Design review of the part built by this model. Coordinates are the model's own, in mm. Face numbers are marked on the shaded views. Coordinates: 2 decimals unless noted, no trailing zeros. Write each loop counter-clockwise with the first axis right and the second up, starting at its lowest first coordinate (ties: lowest second). Pieces come first, ordered by that corner, then holes.
Q1. Take a section at C-C (x = 0). Give the boundary of the cut face in (y, z) (3 decimals), and give its area (3 significant figures).
Q2. Insertion check: pin 1 (3 mm diameter, centred on x = 23.81, y = 0, fed in from +Z). The pin has a flat end and moves straight along its axis. Give the tip position at first contact, or say it passes through.
Q3. Mouldability with a two-part tool opening along X and no side actions: class the marked faces 1, 2, 3 and 4 as pulls with the +X half, pulls with the -X half, needs draft (parallel to the pull), parting line crosses it, or undercut.
Q4. Take a section at B-B (y = 0). Give the boundary of the cut face in (x, z) (3 decimals).
Q5. Take a section at A-A (z = 1.6). Give the boundary of the cut face in (x, y), and give its area (3 significant figures).
Q6. Take a section at D-D (x = 24). Give the boundary of the cut face in (y, z) (3 decimals), and give its area (3 significant figures).
Q7. For probe 1 along Y at (x, z) = (-22, 0.55); probe 2 along X at (y, z) = (-1.5, 0.85); probe 3 along X at (y, z) = (1.75, 1.5), list the stretches that pass through material, from the lowest coordinate up.
Autodesk Inventor part; units mm, degrees
ref_plane "YZ Plane" through (0, 0, 0) normal (1, 0, 0) x (0, 1, 0)
ref_plane "XZ Plane" through (0, 0, 0) normal (0, 1, 0) x (-1, 0, 0)
ref_plane "XY Plane" through (0, 0, 0) normal (0, 0, 1) x (1, 0, 0)
sketch "Sketch1" plane through (0, 0, 0) normal (0, 0, 1) x (1, 0, 0)
  circle A0 centre (0, 0) radius 23.8125 construction
  circle A1 centre (-23.8125, 0) radius 2.4892
  circle A2 centre (23.8125, 0) radius 2.4892
  line L0 (-23.8125, 0) -> (23.8125, 0) construction
  circle A3 centre (0, 0) radius 2.4892
  arc A4 (-25.4861, 5.4113) -> (-25.4861, -5.4113) centre (-23.8125, 0) ccw
  arc A5 (25.4861, -5.4113) -> (25.4861, 5.4113) centre (23.8125, 0) ccw
  line L1 (-25.4861, 5.4113) -> (-3.7524, 12.133)
  line L2 (3.7524, 12.133) -> (25.4861, 5.4113)
  line L3 (25.4861, -5.4113) -> (3.7524, -12.133)
  line L4 (-3.7524, -12.133) -> (-25.4861, -5.4113)
  arc A6 (-3.7524, -12.133) -> (3.7524, -12.133) centre (0, 0) ccw
  arc A7 (3.7524, 12.133) -> (-3.7524, 12.133) centre (0, 0) ccw
  dimension "d0" = 47.625
  dimension "d1" = 4.9784
  dimension "d2" = 3.175
  dimension "d4" = 12.7
  dimension "d5" = 12.7
extrude "Extrusion1" add sketch "Sketch1" along normal blind 3.175
properties part number "Pison Shaft Replacement Screw Plate" material "Thermoplastic Resin"
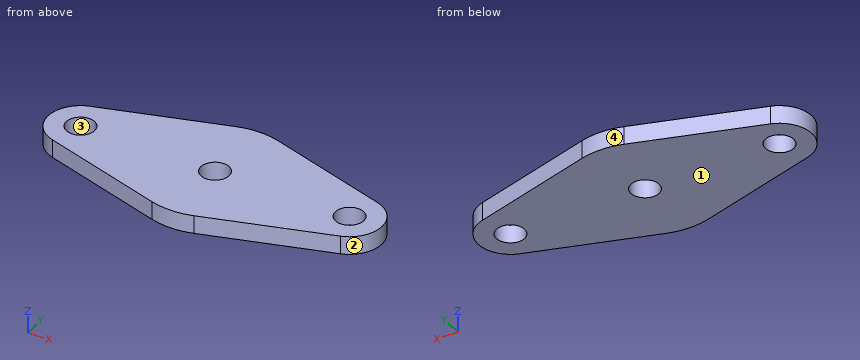
Response:
1. outline: (-12.7, 0) - (-2.489, 0) - (-2.489, 3.175) - (-12.7, 3.175) - close; (2.489, 0) - (12.7, 0) - (12.7, 3.175) - (2.489, 3.175) - close
1. area: 64.8 mm2
2. pin 1: passes through
3. face 1: needs draft
3. face 2: pulls with the +X half
3. face 3: undercut
3. face 4: parting line crosses it
4. outline: (-29.477, 0) - (-26.302, 0) - (-26.302, 3.175) - (-29.477, 3.175) - close; (-21.323, 0) - (-2.489, 0) - (-2.489, 3.175) - (-21.323, 3.175) - close; (2.489, 0) - (21.323, 0) - (21.323, 3.175) - (2.489, 3.175) - close; (26.302, 0) - (29.477, 0) - (29.477, 3.175) - (26.302, 3.175) - close
5. outline: (-25.49, -5.41) - (-3.75, -12.13) arc R12.7 ccw to (3.75, -12.13) - (25.49, -5.41) arc R5.66 ccw to (25.49, 5.41) - (3.75, 12.13) arc R12.7 ccw to (-3.75, 12.13) - (-25.49, 5.41) arc R5.66 ccw to start; hole circle Ø4.98 at (-23.81, 0); hole circle Ø4.98 at (0, 0); hole circle Ø4.98 at (23.81, 0)
5. area: 955 mm2
6. outline: (-5.871, 0) - (-2.482, 0) - (-2.482, 3.175) - (-5.871, 3.175) - close; (2.482, 0) - (5.871, 0) - (5.871, 3.175) - (2.482, 3.175) - close
6. area: 21.5 mm2
7. probe 1: y = -6.49 to -1.71, 1.71 to 6.49
7. probe 2: x = -29.27 to -25.8, -21.83 to -1.99, 1.99 to 21.83, 25.8 to 29.27
7. probe 3: x = -29.2 to -25.58, -22.04 to -1.77, 1.77 to 22.04, 25.58 to 29.2
